Part model, mm, in its own coordinate system. Face numbers are marked on the shaded views. Round coordinates to 2 decimals unless told otherwise and drop trailing zeros. Order: outer loops, then holes, each group sorted by start corner. A loop starts at its lowest first (then second) coordinate and runs counter-clockwise, first axis right, second up. Notation, with made-up numbers: (17.25, -32) -> (68.25, -32) arc R24 cw to (68.25, -5) -> close; hole circle Ø2 at (-15.75, -7.5). An arc over 180 degrees is marked (long way). Answer as a JSON object with one key per item and string values. Group by question number.
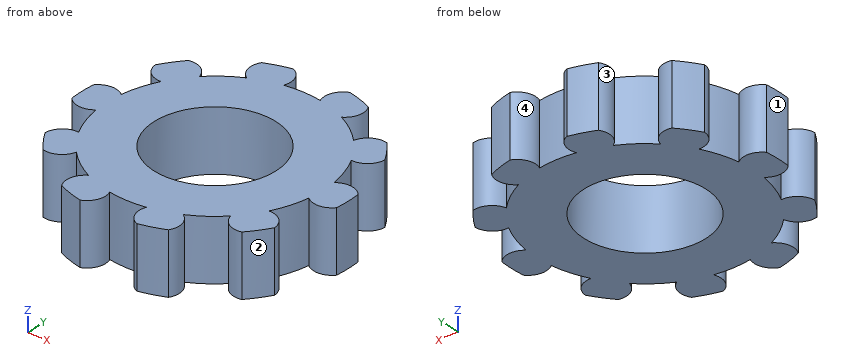
```python
from build123d import *

# Parameters (mm, degrees)
SKETCH1_R           = 13.2
SKETCH1_R_2         = 6
BOSS_EXTRUDE1_DEPTH = 6
CUT_EXTRUDE1_DEPTH  = 7
CIRPATTERN1_COUNT   = 10


with BuildPart() as part:
    # Sketch1 → Boss-Extrude1 (new body)
    with BuildSketch(Plane.XY):
        Circle(SKETCH1_R)
        Circle(SKETCH1_R_2, mode=Mode.SUBTRACT)
    extrude(amount=BOSS_EXTRUDE1_DEPTH)

    # Sketch2 → Cut-Extrude1 (cut, through all)
    with BuildSketch(Plane.XY.offset(6)):
        with BuildLine():
            ThreePointArc((-2.819851171, 12.895287487), (0, 13.2), (2.819851171, 12.895287487))
            ThreePointArc((2.819851171, 12.895287487), (1.826256171, 11.910750525), (1.819851171, 10.512))
            ThreePointArc((1.819851171, 10.512), (0, 10.668364555), (-1.819851171, 10.512))
            ThreePointArc((-1.819851171, 10.512), (-1.826256171, 11.910750525), (-2.819851171, 12.895287487))
        make_face()
    cut_extrude1 = extrude(amount=-CUT_EXTRUDE1_DEPTH, mode=Mode.SUBTRACT)

    # CirPattern1: Cut-Extrude1 ×10 about axis
    cirpattern1_axis = Axis((0, 0, 0), (0, 0, 1))
    for i in range(1, CIRPATTERN1_COUNT):
        add(cut_extrude1.rotate(cirpattern1_axis, i * 360 / CIRPATTERN1_COUNT), mode=Mode.SUBTRACT)


solid = part.part
```
Q1. Drop flat-ended pins along their axis: pin 1 Ø2 at (y, z) = (-5.5, 2) entering from +X; pin 2 Ø1 at (y, z) = (2.5, 5.5) entering from -X. Give the stop position or say it passes through.
Q2. Band-saw the part on A-A (y = 0). List the corners of the cut face in (x, z).
Q3. Band-saw the part on C-C (x = 11). List the corners of the cut face in (y, z).
Q4. Wall check: line 1 (Y direction, x = 0, z = 3.35); line 2 (Y direction, x = -11.75, z = 2.4); line 3 (X direction, y = -7.75, z = 2.1). Give the ranges that are in metal, low to high. Write a range as [from, to].
Q5. Band-saw the part on B-B (x = 0). List the corners of the cut face in (y, z), plus the area to 3 significant figures.
Q6. Two-plate mould, pull along Y, no slides. Class the marked faces 1, 2, 3 and 4: +Y half, -Y half, draft (parallel to the pull), parting line (faces both ways), or undercut.
Completed:
{
 "1": {"pin 1": "x = 11.37", "pin 2": "x = -10.48"},
 "2": {"outline": "(-13.2, 0) -> (-6, 0) -> (-6, 6) -> (-13.2, 6) -> close; (6, 0) -> (13.2, 0) -> (13.2, 6) -> (6, 6) -> close"},
 "3": {"outline": "(-7.3, 0) -> (-5.66, 0) -> (-5.66, 6) -> (-7.3, 6) -> close; (-1.79, 0) -> (1.79, 0) -> (1.79, 6) -> (-1.79, 6) -> close; (5.66, 0) -> (7.3, 0) -> (7.3, 6) -> (5.66, 6) -> close"},
 "4": {"line 1": "[-10.67, -6], [6, 10.67]", "line 2": "[-1.95, 1.95]", "line 3": "[-10.69, -7.76], [-7.33, 7.33], [7.76, 10.69]"},
 "5": {"outline": "(-10.67, 0) -> (-6, 0) -> (-6, 6) -> (-10.67, 6) -> close; (6, 0) -> (10.67, 0) -> (10.67, 6) -> (6, 6) -> close", "area": "56.0 mm2"},
 "6": {"face 1": "parting line", "face 2": "-Y half", "face 3": "undercut", "face 4": "undercut"}
}
